```python
from build123d import *

# Parameters (mm, degrees)
F0_R      = 52.07
F1_DEPTH  = 5.08
F0_R_2    = 55.245
F2_DEPTH  = 30.48
F4_DEPTH  = 21.59
F5_W      = 9.2520020868
F5_H      = 19.05
F6_DEPTH  = 50.8
F7_W      = 9.2520020868
F7_H      = 19.05
F8_DEPTH  = 50.8
F9_W      = 9.2520020868
F9_H      = 19.05
F10_DEPTH = 50.8
F11_W     = 19.05
F11_H     = 9.2520020868
F12_DEPTH = 50.8
F13_W     = 19.05
F13_H     = 9.2520020868
F14_DEPTH = 50.8
F15_W     = 19.05
F15_H     = 9.2520020868
F16_DEPTH = 50.8
F17_W     = 9.2520020868
F17_H     = 19.05
F18_DEPTH = 50.8
F19_W     = 9.2520020868
F19_H     = 19.05
F20_DEPTH = 50.8
F21_W     = 9.2520020868
F21_H     = 19.05
F22_DEPTH = 50.8
F23_W     = 19.05
F23_H     = 9.2520020868
F24_DEPTH = 50.8
F25_W     = 19.05
F25_H     = 9.2520020868
F26_DEPTH = 50.8
F27_W     = 19.05
F27_H     = 9.2520020868
F28_DEPTH = 50.8
F29_W     = 40.64
F29_H     = 38.1
F30_DEPTH = 33.02
F31_DEPTH = 21.59
F33_R     = 2.9464
F34_DEPTH = 1.6256
F32_R     = 11.811
F35_DEPTH = 36.83
F36_W     = 40.64
F36_H     = 38.1
F37_DEPTH = 33.02


with BuildPart() as f1:
    # F0 (on Front) → F1 (new body)
    with BuildSketch(Plane.XZ):
        Circle(F0_R)
    extrude(amount=F1_DEPTH)

    # F0 (on Front) → F2 (join)
    with BuildSketch(Plane.XZ):
        Circle(F0_R_2)
        Circle(F0_R, mode=Mode.SUBTRACT)
    extrude(amount=F2_DEPTH)

    # F3 (on face) → F4 (join)
    with BuildSketch(Plane.XZ.offset(5.08)):
        Polygon((4.5521322669, -17.2840948262), (12.5843095976, -12.6923990675), (17.2445313344, -4.6997852286), (17.2840948262, 4.5521322669), (12.6923990675, 12.5843095976), (4.6997852286, 17.2445313344), (-4.5521322669, 17.2840948262), (-12.5843095976, 12.6923990675), (-17.2445313344, 4.6997852286), (-17.2840948262, -4.5521322669), (-12.6923990675, -12.5843095976), (-4.6997852286, -17.2445313344), align=None)
    extrude(amount=F4_DEPTH)

    # F5 (on face) → F6 (cut)
    with BuildSketch(Plane(origin=(8.696092148, 0, 14.914420466), x_dir=(0.8638793813, 0, -0.5036987339), z_dir=(0.5036987339, 0, 0.8638793813))):
        with Locations((0, -17.145)):
            Rectangle(F5_W, F5_H)
    extrude(amount=F6_DEPTH, mode=Mode.SUBTRACT)

    # F7 (on face) → F8 (cut)
    with BuildSketch(Plane(origin=(0.0738264808, 0, 17.2643130803), x_dir=(0.999990857, 0, -0.0042762087), z_dir=(0.0042762087, 0, 0.999990857))):
        with Locations((0, -17.145)):
            Rectangle(F7_W, F7_H)
    extrude(amount=F8_DEPTH, mode=Mode.SUBTRACT)

    # F9 (on face) → F10 (cut)
    with BuildSketch(Plane(origin=(-8.5682209323, 0, 14.9882469469), x_dir=(0.86815559, 0, 0.4962921231), z_dir=(-0.4962921231, 0, 0.86815559))):
        with Locations((0, -17.145)):
            Rectangle(F9_W, F9_H)
    extrude(amount=F10_DEPTH, mode=Mode.SUBTRACT)

    # F11 (on face) → F12 (cut)
    with BuildSketch(Plane(origin=(-14.914420466, 0, 8.696092148), x_dir=(0, -1, 0), z_dir=(-0.8638793813, 0, 0.5036987339))):
        with Locations((17.145, 0)):
            Rectangle(F11_W, F11_H)
    extrude(amount=F12_DEPTH, mode=Mode.SUBTRACT)

    # F13 (on face) → F14 (cut)
    with BuildSketch(Plane(origin=(-17.2643130803, 0, 0.0738264808), x_dir=(0, -1, 0), z_dir=(-0.999990857, 0, 0.0042762087))):
        with Locations((17.145, 0)):
            Rectangle(F13_W, F13_H)
    extrude(amount=F14_DEPTH, mode=Mode.SUBTRACT)

    # F15 (on face) → F16 (cut)
    with BuildSketch(Plane(origin=(-14.9882469469, 0, -8.5682209323), x_dir=(0, -1, 0), z_dir=(-0.86815559, 0, -0.4962921231))):
        with Locations((17.145, 0)):
            Rectangle(F15_W, F15_H)
    extrude(amount=F16_DEPTH, mode=Mode.SUBTRACT)

    # F17 (on face) → F18 (cut)
    with BuildSketch(Plane(origin=(-8.696092148, 0, -14.914420466), x_dir=(0.8638793813, 0, -0.5036987339), z_dir=(-0.5036987339, 0, -0.8638793813))):
        with Locations((0, 17.145)):
            Rectangle(F17_W, F17_H)
    extrude(amount=F18_DEPTH, mode=Mode.SUBTRACT)

    # F19 (on face) → F20 (cut)
    with BuildSketch(Plane(origin=(-0.0738264808, 0, -17.2643130803), x_dir=(0.999990857, 0, -0.0042762087), z_dir=(-0.0042762087, 0, -0.999990857))):
        with Locations((0, 17.145)):
            Rectangle(F19_W, F19_H)
    extrude(amount=F20_DEPTH, mode=Mode.SUBTRACT)

    # F21 (on face) → F22 (cut)
    with BuildSketch(Plane(origin=(8.5682209323, 0, -14.9882469469), x_dir=(0.86815559, 0, 0.4962921231), z_dir=(0.4962921231, 0, -0.86815559))):
        with Locations((0, 17.145)):
            Rectangle(F21_W, F21_H)
    extrude(amount=F22_DEPTH, mode=Mode.SUBTRACT)

    # F23 (on face) → F24 (cut)
    with BuildSketch(Plane(origin=(14.914420466, 0, -8.696092148), x_dir=(0, 1, 0), z_dir=(0.8638793813, 0, -0.5036987339))):
        with Locations((-17.145, 0)):
            Rectangle(F23_W, F23_H)
    extrude(amount=F24_DEPTH, mode=Mode.SUBTRACT)

    # F25 (on face) → F26 (cut)
    with BuildSketch(Plane(origin=(17.2643130803, 0, -0.0738264808), x_dir=(0, 1, 0), z_dir=(0.999990857, 0, -0.0042762087))):
        with Locations((-17.145, 0)):
            Rectangle(F25_W, F25_H)
    extrude(amount=F26_DEPTH, mode=Mode.SUBTRACT)

    # F27 (on face) → F28 (cut)
    with BuildSketch(Plane(origin=(14.9882469469, 0, 8.5682209323), x_dir=(0, 1, 0), z_dir=(0.86815559, 0, 0.4962921231))):
        with Locations((-17.145, 0)):
            Rectangle(F27_W, F27_H)
    extrude(amount=F28_DEPTH, mode=Mode.SUBTRACT)

    # F29 (on face) → F30 (join)
    with BuildSketch(Plane.XZ):
        with Locations((0.0789208158, 0.021902828)):
            Rectangle(F29_W, F29_H)
    extrude(amount=-F30_DEPTH)

    # F31 (cut): a face of the model
    f31_faces = [f1.faces().sort_by_distance(p)[0] for p in [
        (0, -26.67, 0),
    ]]
    extrude(f31_faces, amount=-F31_DEPTH, mode=Mode.SUBTRACT)

    # F33 (on face) → F34 (cut)
    with BuildSketch(Plane.XZ.offset(5.08)):
        Circle(F33_R)
    extrude(amount=-F34_DEPTH, mode=Mode.SUBTRACT)

    # F32 (on face) → F35 (cut)
    with BuildSketch(Plane(origin=(0, 33.02, 0), x_dir=(-1, 0, 0), z_dir=(0, 1, 0))):
        Circle(F32_R)
    extrude(amount=-F35_DEPTH, mode=Mode.SUBTRACT)

    # F36 (on face) → F37 (cut)
    with BuildSketch(Plane(origin=(0, 33.02, 0), x_dir=(-1, 0, 0), z_dir=(0, 1, 0))):
        with Locations((-0.0789208158, 0.021902828)):
            Rectangle(F36_W, F36_H)
        Polygon((17.6803887808, 0), (8.8401943904, -15.311665833), (-8.8401943904, -15.311665833), (-17.6803887808, 0), (-8.8401943904, 15.311665833), (8.8401943904, 15.311665833), align=None, mode=Mode.SUBTRACT)
    extrude(amount=-F37_DEPTH, mode=Mode.SUBTRACT)


solid = f1.part
```
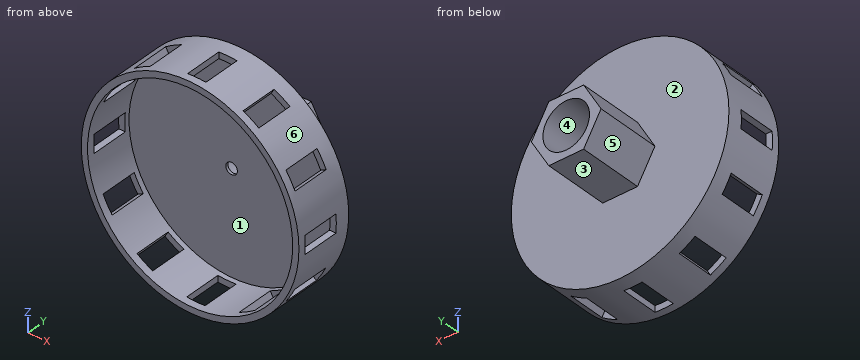
The model under review builds one solid part; all positions refer to its coordinate system, in mm. Face numbers are marked on the shaded views. A direction names the side the tool comes from. Round coordinates to 2 decimals unless told otherwise and drop trailing zeros. Write each loop counter-clockwise with the first axis right and the second up, starting at its lowest first coordinate (ties: lowest second). Pieces come first, ordered by that corner, then holes.
(1) We need section D-D on x = -26.5. Give the boundary of the cut face in (y, z).
(2) We need section B-B on x = 0. Give the boundary of the cut face in (y, z) (3 decimals).
(3) We need section A-A on y = 24.5. Give the boundary of the cut face in (x, z).
(4) We need section C-C on y = -14. Give the number of separate pieces and of enclosed holes in the cut face, and give its area (3 significant figures).
(5) Mouldability with a two-part tool opening along Z and no side actions: class the marked faces 4, 5 and 6 as +Z half, -Z half, draft (parallel to the pull), parting line (faces both ways), or undercut.
(6) Machinability: for the marked faces 1, 2 and 3, which of the approach directions +Z, -Z, +X, -X, +Y, -Y give a long, thin tool a straight path to every point of the face, cutting with its end or side? Answer none if there is none.
(7) Wall thickness on L1, parallel to Z at x = 0, y = 23; L2, parallel to Y at x = -23, z = -25; L3, parallel to Z at x = 5, y = 8: over which ranges is each line inside the solid? List them lowest first.
(8) Insertion check: pin 1 (8 mm diameter, centred on x = 25.5, z = -45, fed in from +Y); pin 2 (6 mm diameter, centred on y = -0.5, z = 43, fed in from +X); pin 3 (5 mm diameter, centred on y = -8.5, z = -23.5, fed in from +X); pin 4 (2 mm diameter, centred on y = 25, z = -17, fed in from -X). Each pin has a flat end and moves straight along its axis. Give the tip position at first contact, or say it passes through.
Findings below:
1. outline: (-30.48, -48.47) - (-26.67, -48.47) - (-26.67, -44.82) - (-30.48, -44.82) - close; (-30.48, 44.82) - (-26.67, 44.82) - (-26.67, 48.47) - (-30.48, 48.47) - close; (-7.62, -48.47) - (0, -48.47) - (0, 48.47) - (-7.62, 48.47) - (-7.62, 44.82) - (-5.08, 44.82) - (-5.08, -44.82) - (-7.62, -44.82) - close
2. outline: (-30.48, -55.245) - (-26.67, -55.245) - (-26.67, -52.07) - (-30.48, -52.07) - close; (-30.48, 52.07) - (-26.67, 52.07) - (-26.67, 55.245) - (-30.48, 55.245) - close; (-7.62, -55.245) - (0, -55.245) - (0, -15.312) - (33.02, -15.312) - (33.02, -11.811) - (-3.81, -11.811) - (-3.81, -2.946) - (-5.08, -2.946) - (-5.08, -52.07) - (-7.62, -52.07) - close; (-7.62, 52.07) - (-5.08, 52.07) - (-5.08, 2.946) - (-3.81, 2.946) - (-3.81, 11.811) - (33.02, 11.811) - (33.02, 15.312) - (0, 15.312) - (0, 55.245) - (-7.62, 55.245) - close
3. outline: (-17.68, 0) - (-8.84, -15.31) - (8.84, -15.31) - (17.68, 0) - (8.84, 15.31) - (-8.84, 15.31) - close; hole circle Ø23.62 at (0, 0)
4. separate pieces: 12
4. enclosed holes: 0
4. area: 717 mm2
5. face 4: undercut
5. face 5: -Z half
5. face 6: parting line
6. face 1: -Y
6. face 2: +Y
6. face 3: -Z, +X, -X, +Y
7. L1: z = -15.31 to -11.81, 11.81 to 15.31
7. L2: y = -5.08 to 0
7. L3: z = -15.31 to -10.7, 10.7 to 15.31
8. pin 1: stops at y = 0
8. pin 2: stops at x = 38.11
8. pin 3: stops at x = 51.1
8. pin 4: passes through
